Check sheet for the modelled part. Datum: model origin and axes. Units: mm. Face numbers are marked on the shaded views. A direction names the side the tool comes from. Round coordinates to 2 decimals unless told otherwise and drop trailing zeros. Order: outer loops, then holes, each group sorted by start corner. A loop starts at its lowest first (then second) coordinate and runs counter-clockwise, first axis right, second up. Notation, with made-up numbers: M 15.25,39.5 L 26.25,39.5 A15 ccw 26.25,46.5 Z; hole C -7,-11.75 d5. An arc over 180 degrees is marked long. One line per item, written item: value. Start each with the question number.
(1) Cross-section at B-B, the plane y = 7.44. Enter the section's corners in (x, z), and give its area (3 significant figures).
(2) Cross-section at D-D, the plane y = 13.5. Enter the section's corners in (x, z).
(3) Cross-section at A-A, the plane x = 0. Enter the section's corners in (y, z).
(4) Access from +Z, -Z, +X, -X, +Y, -Y to the whole of each face (thin tool, end or side, straight path). Record for the marked faces 5, 6, 7 and 8.
(5) Thickness scan on L1, parallel to Y at x = -20, z = 42; L2, parallel to X at y = 9, z = 42.5; L3, parallel to Y at x = -16, z = 40. Record the ranges inside material, lowest first.
(6) Release check for a two-part mould opening along Y. For the marked faces 1, 2, 3 and 4 record: released by +Y, released by -Y, zero draft, split by the parting line, or undercut.
(7) Depth check by flat-ended pin: pin 1 Ø3.5 at (x, z) = (-12.5, 40) entering from +Y; pin 2 Ø7 at (x, y) = (0, 8) entering from -Z; pin 3 Ø0.6 at (y, z) = (4, 44.5) entering from +X; pin 4 Ø4.5 at (x, y) = (-12, 15) entering from +Z. Enter the tip coordinate at first touch or a pass-through.
(8) Cross-section at C-C, the plane z = 42.5. Enter the section's corners in (x, y).
from build123d import *
from OCP.BRepFilletAPI import BRepFilletAPI_MakeChamfer

# Parameters (mm, degrees)
AUFSATZ_LINEAR_AUSTRAGEN1_DEPTH    = 6.1
AUFSATZ_LINEAR_AUSTRAGEN1_2_DEPTH  = 6.1
SKIZZE2_W                          = 6
SKIZZE2_H                          = 10.88
SCHNITT_LINEAR_AUSTRAGEN1_DEPTH    = 6.1
SKIZZE3_R                          = 2.65
SKIZZE3_W                          = 6.1
SKIZZE3_H                          = 4.12
AUFSATZ_LINEAR_AUSTRAGEN2_DEPTH    = 2.19
SKIZZE4_R                          = 2.65
AUFSATZ_LINEAR_AUSTRAGEN3_DEPTH    = 4.81
SKIZZE5_R                          = 2.65
AUFSATZ_LINEAR_AUSTRAGEN4_DEPTH    = 0.19
FASE1_SIZE                         = 5
FASE1_SIZE2                        = 8.660254038
FASE2_SIZE                         = 2
FASE2_SIZE2                        = 1.154700538
SCHNITT_LINEAR_START               = -4
SCHNITT_LINEAR_AUSTRAGEN3_DEPTH    = 2.5
SCHNITT_LINEAR_AUSTRAGEN4_REACH    = 67.9
SKIZZE12_W                         = 5
SKIZZE12_H                         = 6.1
K_RPER_VERSCHIEBEN_KOPIEREN1_ANGLE = 90


with BuildPart() as part:
    # Skizze1 → Aufsatz-Linear austragen1 (new body)
    with BuildSketch(Plane.XY):
        Polygon((0, 0), (0, 9.44), (0, 10.88), (-6, 10.88), (-6, 0), align=None)
    extrude(amount=AUFSATZ_LINEAR_AUSTRAGEN1_DEPTH)

    # Skizze2 → Schnitt-Linear austragen1 (cut)
    with BuildSketch(Plane.XY.offset(6.1)):
        with Locations((-3, 5.44)):
            Rectangle(SKIZZE2_W, SKIZZE2_H)
    extrude(amount=-SCHNITT_LINEAR_AUSTRAGEN1_DEPTH, mode=Mode.SUBTRACT)


with BuildPart() as body_2:
    # Skizze1 → Aufsatz-Linear austragen1 2 (new body)
    with BuildSketch(Plane.XY):
        with BuildLine():
            Line((-7.05, 10.19), (-7.05, 10.69))
            ThreePointArc((-7.05, 10.69), (-7.105649712, 10.824350288), (-7.24, 10.88))
            Line((-7.24, 10.88), (-9.24, 10.88))
            Line((-9.24, 10.88), (-9.24, 0))
            Line((-9.24, 0), (-7.24, 0))
            ThreePointArc((-7.24, 0), (-7.105649712, 0.055649712), (-7.05, 0.19))
            Line((-7.05, 0.19), (-7.05, 0.69))
            ThreePointArc((-7.05, 0.69), (-7.105649712, 0.824350288), (-7.24, 0.88))
            ThreePointArc((-7.24, 0.88), (-7.8, 1.44), (-7.24, 2))
            ThreePointArc((-7.24, 2), (-7.105649712, 2.055649712), (-7.05, 2.19))
            Line((-7.05, 2.19), (-7.05, 2.69))
            ThreePointArc((-7.05, 2.69), (-7.105649712, 2.824350288), (-7.24, 2.88))
            ThreePointArc((-7.24, 2.88), (-7.8, 3.44), (-7.24, 4))
            ThreePointArc((-7.24, 4), (-7.105649712, 4.055649712), (-7.05, 4.19))
            Line((-7.05, 4.19), (-7.05, 4.69))
            ThreePointArc((-7.05, 4.69), (-7.105649712, 4.824350288), (-7.24, 4.88))
            ThreePointArc((-7.24, 4.88), (-7.8, 5.44), (-7.24, 6))
            ThreePointArc((-7.24, 6), (-7.105649712, 6.055649712), (-7.05, 6.19))
            Line((-7.05, 6.19), (-7.05, 6.69))
            ThreePointArc((-7.05, 6.69), (-7.105649712, 6.824350288), (-7.24, 6.88))
            ThreePointArc((-7.24, 6.88), (-7.8, 7.44), (-7.24, 8))
            ThreePointArc((-7.24, 8), (-7.105649712, 8.055649712), (-7.05, 8.19))
            Line((-7.05, 8.19), (-7.05, 8.69))
            ThreePointArc((-7.05, 8.69), (-7.105649712, 8.824350288), (-7.24, 8.88))
            ThreePointArc((-7.24, 8.88), (-7.8, 9.44), (-7.24, 10))
            ThreePointArc((-7.24, 10), (-7.105649712, 10.055649712), (-7.05, 10.19))
        make_face()
    extrude(amount=AUFSATZ_LINEAR_AUSTRAGEN1_2_DEPTH)

    # Skizze3 → Aufsatz-Linear austragen2 (add)
    # profile 1 of 2: a face of its own
    with BuildSketch(Plane.ZY.offset(9.24)):
        Polygon((-13, -2), (0, -2), (0, 13.88), (0, 18), (-13, 18), align=None)
        with Locations((-4, 8)):
            Circle(SKIZZE3_R, mode=Mode.SUBTRACT)
    # profile 2 of 2: a face of its own
    with BuildSketch(Plane.ZY.offset(9.24)):
        with Locations((3.05, 15.94)):
            Rectangle(SKIZZE3_W, SKIZZE3_H)
    extrude(amount=-AUFSATZ_LINEAR_AUSTRAGEN2_DEPTH)

    # Skizze4 → Aufsatz-Linear austragen3 (add)
    # profile 1 of 2: a face of its own
    with BuildSketch(Plane.ZY.offset(9.24)):
        Polygon((24.1, 18), (6.1, 18), (6.1, 13.88), (6.1, 10.88), (6.1, 0), (6.1, -2), (24.1, -2), align=None)
        with Locations((16.1, 8)):
            Circle(SKIZZE4_R, mode=Mode.SUBTRACT)
    # profile 2 of 2: a face of its own
    with BuildSketch(Plane.ZY.offset(9.24)):
        Polygon((6.1, 0), (6.1, 10.88), (0, 10.88), (0, 13.88), (6.1, 13.88), (6.1, 18), (-13, 18), (-13, -2), (0, -2), (0, 0), align=None)
        with Locations((-4, 8)):
            Circle(SKIZZE4_R, mode=Mode.SUBTRACT)
    extrude(amount=AUFSATZ_LINEAR_AUSTRAGEN3_DEPTH)

    # Skizze5 → Aufsatz-Linear austragen4 (add)
    with BuildSketch(Plane(origin=(-9.24, 0, 0), x_dir=(0, 0, -1), z_dir=(1, 0, 0))):
        Polygon((-6.1, 13.88), (-6.1, 18), (-24.1, 18), (-24.1, -2), (-6.1, -2), (-6.1, 0), (-6.1, 10.88), align=None)
        with Locations(Location((-16.1, 8, 0), (0, 0, 180))):
            Circle(SKIZZE5_R, mode=Mode.SUBTRACT)
    extrude(amount=AUFSATZ_LINEAR_AUSTRAGEN4_DEPTH)

    # Fase1: one chamfer whose edges measure the first distance from different faces: ONE call of the kernel's chamfer builder (chamfer() names one face for all edges)
    fase1_edges_1 = [body_2.edges().sort_by_distance(p)[0] for p in [
        (-11.645, -2, 24.1),
        (-11.645, 18, 24.1),
    ]]
    fase1_side_1 = [body_2.faces().sort_by_distance(p)[0] for p in [
        (-11.645, 8, 24.1),
    ]]
    fase1_edges_2 = [body_2.edges().sort_by_distance(p)[0] for p in [
        (-10.55, -2, -13),
        (-10.55, 18, -13),
    ]]
    fase1_side_2 = [body_2.faces().sort_by_distance(p)[0] for p in [
        (-10.55, 8, -13),
    ]]
    fase1 = BRepFilletAPI_MakeChamfer(body_2.part.solid().wrapped)
    for e in fase1_edges_1:
        fase1.Add(FASE1_SIZE, FASE1_SIZE2, e.wrapped, fase1_side_1[0].wrapped)  # the first distance lies on this face
    for e in fase1_edges_2:
        fase1.Add(FASE1_SIZE, FASE1_SIZE2, e.wrapped, fase1_side_2[0].wrapped)  # the first distance lies on this face
    add(Compound.cast(fase1.Shape()), mode=Mode.REPLACE)

    # Fase2: one chamfer whose edges measure the first distance from different faces: ONE call of the kernel's chamfer builder (chamfer() names one face for all edges)
    fase2_edges_1 = [body_2.edges().sort_by_distance(p)[0] for p in [
        (-14.05, -2, 10.769872981),
    ]]
    fase2_side_1 = [body_2.faces().sort_by_distance(p)[0] for p in [
        (-11.645, -2, 10.769872981),
    ]]
    fase2_edges_2 = [body_2.edges().sort_by_distance(p)[0] for p in [
        (-14.05, 10.88, 3.05),
    ]]
    fase2_side_2 = [body_2.faces().sort_by_distance(p)[0] for p in [
        (-11.645, 10.88, 3.05),
    ]]
    fase2_edges_3 = [body_2.edges().sort_by_distance(p)[0] for p in [
        (-14.05, 13.88, 3.05),
    ]]
    fase2_side_3 = [body_2.faces().sort_by_distance(p)[0] for p in [
        (-10.55, 13.88, 3.05),
    ]]
    fase2_edges_4 = [body_2.edges().sort_by_distance(p)[0] for p in [
        (-14.05, 18, 5.55),
    ]]
    fase2_side_4 = [body_2.faces().sort_by_distance(p)[0] for p in [
        (-10.939880768, 18, 4.735948766),
    ]]
    fase2_edges_5 = [body_2.edges().sort_by_distance(p)[0] for p in [
        (-14.05, 8, 24.1),
    ]]
    fase2_side_5 = [body_2.faces().sort_by_distance(p)[0] for p in [
        (-11.645, 8, 24.1),
    ]]
    fase2_edges_6 = [body_2.edges().sort_by_distance(p)[0] for p in [
        (-14.05, 8, -13),
    ]]
    fase2_side_6 = [body_2.faces().sort_by_distance(p)[0] for p in [
        (-10.55, 8, -13),
    ]]
    fase2_edges_7 = [body_2.edges().sort_by_distance(p)[0] for p in [
        (-14.05, -2, -2.169872981),
    ]]
    fase2_side_7 = [body_2.faces().sort_by_distance(p)[0] for p in [
        (-10.55, -2, -2.169872981),
    ]]
    fase2_edges_8 = [body_2.edges().sort_by_distance(p)[0] for p in [
        (-14.05, 0.5, -8.669872981),
    ]]
    fase2_side_8 = [body_2.faces().sort_by_distance(p)[0] for p in [
        (-10.55, 0.5, -8.669872981),
    ]]
    fase2_edges_9 = [body_2.edges().sort_by_distance(p)[0] for p in [
        (-14.05, 0.5, 19.769872981),
    ]]
    fase2_side_9 = [body_2.faces().sort_by_distance(p)[0] for p in [
        (-11.645, 0.5, 19.769872981),
    ]]
    fase2_edges_10 = [body_2.edges().sort_by_distance(p)[0] for p in [
        (-14.05, 15.5, 19.769872981),
    ]]
    fase2_side_10 = [body_2.faces().sort_by_distance(p)[0] for p in [
        (-11.645, 15.5, 19.769872981),
    ]]
    fase2_edges_11 = [body_2.edges().sort_by_distance(p)[0] for p in [
        (-14.05, 15.5, -8.669872981),
    ]]
    fase2_side_11 = [body_2.faces().sort_by_distance(p)[0] for p in [
        (-10.55, 15.5, -8.669872981),
    ]]
    fase2 = BRepFilletAPI_MakeChamfer(body_2.part.solid().wrapped)
    for e in fase2_edges_1:
        fase2.Add(FASE2_SIZE, FASE2_SIZE2, e.wrapped, fase2_side_1[0].wrapped)  # the first distance lies on this face
    for e in fase2_edges_2:
        fase2.Add(FASE2_SIZE, FASE2_SIZE2, e.wrapped, fase2_side_2[0].wrapped)  # the first distance lies on this face
    for e in fase2_edges_3:
        fase2.Add(FASE2_SIZE, FASE2_SIZE2, e.wrapped, fase2_side_3[0].wrapped)  # the first distance lies on this face
    for e in fase2_edges_4:
        fase2.Add(FASE2_SIZE, FASE2_SIZE2, e.wrapped, fase2_side_4[0].wrapped)  # the first distance lies on this face
    for e in fase2_edges_5:
        fase2.Add(FASE2_SIZE, FASE2_SIZE2, e.wrapped, fase2_side_5[0].wrapped)  # the first distance lies on this face
    for e in fase2_edges_6:
        fase2.Add(FASE2_SIZE, FASE2_SIZE2, e.wrapped, fase2_side_6[0].wrapped)  # the first distance lies on this face
    for e in fase2_edges_7:
        fase2.Add(FASE2_SIZE, FASE2_SIZE2, e.wrapped, fase2_side_7[0].wrapped)  # the first distance lies on this face
    for e in fase2_edges_8:
        fase2.Add(FASE2_SIZE, FASE2_SIZE2, e.wrapped, fase2_side_8[0].wrapped)  # the first distance lies on this face
    for e in fase2_edges_9:
        fase2.Add(FASE2_SIZE, FASE2_SIZE2, e.wrapped, fase2_side_9[0].wrapped)  # the first distance lies on this face
    for e in fase2_edges_10:
        fase2.Add(FASE2_SIZE, FASE2_SIZE2, e.wrapped, fase2_side_10[0].wrapped)  # the first distance lies on this face
    for e in fase2_edges_11:
        fase2.Add(FASE2_SIZE, FASE2_SIZE2, e.wrapped, fase2_side_11[0].wrapped)  # the first distance lies on this face
    add(Compound.cast(fase2.Shape()), mode=Mode.REPLACE)

    # Skizze11 → Schnitt-Linear austragen3 (cut)
    with BuildSketch(Plane.XZ.offset(2).offset(SCHNITT_LINEAR_START)):
        with BuildLine():
            Line((-14.05, 7.6), (-14.05, 6.1))
            ThreePointArc((-14.05, 6.1), (-12.989339828, 5.660660172), (-12.55, 4.6))
            Line((-12.55, 4.6), (-12.55, 1.5))
            ThreePointArc((-12.55, 1.5), (-12.989339828, 0.439339828), (-14.05, 0))
            Line((-14.05, 0), (-14.05, -1.5))
            ThreePointArc((-14.05, -1.5), (-11.928679656, -0.621320344), (-11.05, 1.5))
            Line((-11.05, 1.5), (-11.05, 4.6))
            ThreePointArc((-11.05, 4.6), (-11.928679656, 6.721320344), (-14.05, 7.6))
        make_face()
    extrude(amount=-SCHNITT_LINEAR_AUSTRAGEN3_DEPTH, mode=Mode.SUBTRACT)


with BuildPart() as body_2_2:
    # Spiegeln1: mirrored copy
    add(body_2.part.mirror(Plane(origin=(-63.197479165, -24.924466517, 24.1), x_dir=(1, 0, 0), z_dir=(0, 0, 1))))

    # Schnitt-Linear austragen4: up to this plane
    schnitt_linear_austragen4_end = Plane(origin=(-14.05, 15.034700538, 42.1), z_dir=(0.4999999999999981, 0.8660254037844397, 0))
    # Skizze12 → Schnitt-Linear austragen4 (cut, up to the surface)
    with BuildSketch(Plane(origin=(0, 18, 0), x_dir=(1, 0, 0), z_dir=(0, 1, 0)), mode=Mode.PRIVATE) as schnitt_linear_austragen4_sk1:
        with Locations((-9.55, -45.15)):
            Rectangle(SKIZZE12_W, SKIZZE12_H)
    schnitt_linear_austragen4_tool1 = split(extrude(schnitt_linear_austragen4_sk1.sketch, amount=-SCHNITT_LINEAR_AUSTRAGEN4_REACH, mode=Mode.PRIVATE), bisect_by=schnitt_linear_austragen4_end, keep=Keep.BOTH, mode=Mode.PRIVATE)
    add(schnitt_linear_austragen4_tool1.solids().sort_by_distance((-9.55, 18, 45.15))[0], mode=Mode.SUBTRACT)


with BuildPart() as body_2_2_1:
    # Körper-Verschieben/Kopieren1: moved
    add(body_2_2.part.rotate(Axis((-10.55, 0, 42.65), (0, -1, 0)), K_RPER_VERSCHIEBEN_KOPIEREN1_ANGLE))


solid = body_2_2_1.part
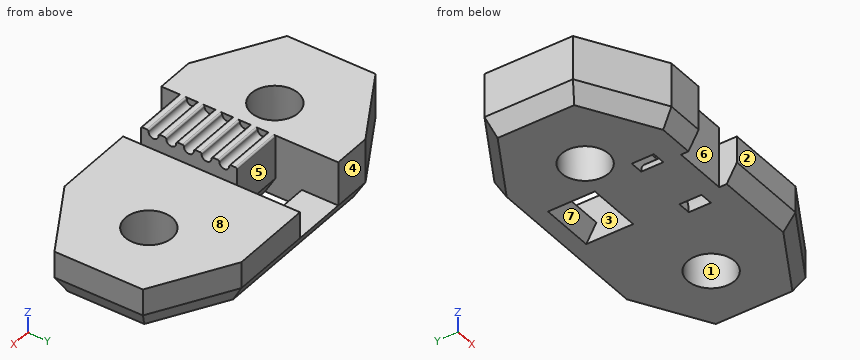
Values found:
1. outline: M -29.1,41.15 L -27.95,39.15 L -22.69,39.15 L -22.69,46.15 L -29.1,46.15 Z; M -17.51,39.15 L -2.59,39.15 L -2.59,44.15 L -10,44.15 L -10,45.4 L -16.1,45.4 L -16.1,46.15 L -17.51,46.15 Z; M 2.59,39.15 L 6.85,39.15 L 8,41.15 L 8,44.15 L 2.59,44.15 Z
1. area: 155 mm^2
2. outline: M -28.23,41.15 L -25.92,39.15 L -16.1,39.15 L -16.1,46.15 L -28.23,46.15 Z; M -10,39.15 L 4.82,39.15 L 7.13,41.15 L 7.13,44.15 L -10,44.15 Z
3. outline: M -1.62,41.15 L -0.29,39.15 L 5.35,39.15 L 5.35,44.15 L -1.62,44.15 Z; M 10.65,39.15 L 16.29,39.15 L 17.62,41.15 L 17.62,44.15 L 10.65,44.15 Z
4. face 5: +Z, -Z, +Y
4. face 6: +Z, -Z, -Y
4. face 7: -Z
4. face 8: +Z, +X, +Y, -Y
5. L1: -2 to 5.35, 10.65 to 18
5. L2: -29.1 to -22.55, -17.65 to -2.45, 2.45 to 8
5. L3: 0 to 2, 4.5 to 10.22, 14.54 to 17.34
6. face 1: undercut
6. face 2: released by -Y
6. face 3: undercut
6. face 4: released by +Y
7. pin 1: y = 18
7. pin 2: z = 39.15
7. pin 3: x = -10
7. pin 4: z = 44.15
8. outline: M -29.1,3 L -20.44,-2 L -16.1,-2 L -16.1,0 L -10,0 L -10,-2 L -0.66,-2 L 8,3 L 8,13 L -0.66,18 L -10,18 L -10,10.88 L -16.1,10.88 L -16.1,18 L -20.44,18 L -29.1,13 Z; hole C -20.1,8 d5.3; hole C 0,8 d5.3
